CAD build for the part. Positions are in the model's coordinates, mm. Coordinates: 2 decimals unless noted, no trailing zeros. Write each loop counter-clockwise with the first axis right and the second up, starting at its lowest first coordinate (ties: lowest second). Pieces come first, ordered by that corner, then holes. Notation, with made-up numbers: (42.25, 50.25) - (89.25, 50.25) arc R18 cw to (89.25, 85.25) - close; hole circle Ø4 at (-29.5, -27.5). An arc over 180 degrees is marked (long way). One line per question, with ' | ' between items. Start each with the question number.
1. Band-saw the part on D-D, the plane z = -5.5. Write the cut outline in (x, y), then the cut area to 3 significant figures.
2. Flat gauge pins, fed straight in: P1, Ø5.5, axis at y = 97.47, z = 3.94, coming from the +X side; P2, Ø1.5, axis at x = 30.5, z = -56, coming from the +Y side; P3, Ø1.5, axis at x = 30.5, y = 98, coming from the +Z side; P4, Ø10, axis at y = 125.5, z = -1, coming from the +X side. Where does each tip first touch, or does it go through?
3. Band-saw the part on A-A, the plane y = 42. Write the cut outline in (x, z).
4. Band-saw the part on C-C, the plane z = -22.5. Write the cut outline in (x, y), then the cut area to 3 significant figures.
5. Two-plate mould, pull along Z, no slides. Class faces 1 (the cylindrical face through (29.786, 108.104, -65.421)), 2 (the cylindrical face through (30.48, 139.74, -30.23)), 3 (the flat face through (30.48, 131, -54.37)): +Z half, -Z half, draft (parallel to the pull), parting line (faces both ways), or undercut.
6. Probe line 1 (Z direction, x = 29.4, y = 42); line 2 (Z direction, x = 30.9, y = 85); line 3 (Y direction, x = 29.45, z = 22.5). List the from-to ranges inside material, lowest first.
7. Band-saw the part on B-B, the plane x = 29.6. Give the number of separate pieces and of enclosed holes in the cut face, then the cut area to 3 significant figures.
from build123d import *

# Parameters (mm, degrees)
BOSS_EXTRUDE1_DEPTH                            = 3
CSK_FOR_M3_FLAT_HEAD_MACHINE_SCREW1_AT_2_COUNT = 2
CSK_FOR_M3_FLAT_HEAD_MACHINE_SCREW1_AT_2_PITCH = 24.36335345
CSK_FOR_M3_FLAT_HEAD_MACHINE_SCREW1_AT_3_COUNT = 2
CSK_FOR_M3_FLAT_HEAD_MACHINE_SCREW1_AT_3_PITCH = 69.5
CSK_FOR_M3_FLAT_HEAD_MACHINE_SCREW1_AT_4_COUNT = 2
CSK_FOR_M3_FLAT_HEAD_MACHINE_SCREW1_AT_4_PITCH = 73.646608824
CSK_FOR_M3_FLAT_HEAD_MACHINE_SCREW1_AT_5_COUNT = 2
CSK_FOR_M3_FLAT_HEAD_MACHINE_SCREW1_AT_5_PITCH = 56.579922425
CSK_FOR_M3_FLAT_HEAD_MACHINE_SCREW1_AT_6_COUNT = 2
CSK_FOR_M3_FLAT_HEAD_MACHINE_SCREW1_AT_6_PITCH = 38.581652039
CSK_FOR_M3_FLAT_HEAD_MACHINE_SCREW1_AT_7_COUNT = 2
CSK_FOR_M3_FLAT_HEAD_MACHINE_SCREW1_AT_7_PITCH = 110.143173396
CSK_FOR_M3_FLAT_HEAD_MACHINE_SCREW1_AT_8_COUNT = 2
CSK_FOR_M3_FLAT_HEAD_MACHINE_SCREW1_AT_8_PITCH = 79.535664399


with BuildPart() as part:
    # Sketch2 → Boss-Extrude1 (new body)
    with BuildSketch(Plane(origin=(29, 0, 0), x_dir=(0, 0, -1), z_dir=(1, 0, 0))):
        with BuildLine():
            Line((-16.691511003, 108.816260881), (16.610141275, 134.506640075))
            ThreePointArc((16.610141275, 134.506640075), (30.439693581, 139.756494337), (44.856843921, 136.445412513))
            Line((44.856843921, 136.445412513), (64.147238229, 125.399811115))
            ThreePointArc((64.147238229, 125.399811115), (67.359474123, 122.47213667), (69.026291478, 118.458228724))
            Line((69.026291478, 118.458228724), (76.03531425, 78.708085309))
            ThreePointArc((76.03531425, 78.708085309), (75.841855651, 74.366160521), (73.824664919, 70.516397068))
            Line((73.824664919, 70.516397068), (59.475441909, 53.539223516))
            ThreePointArc((59.475441909, 53.539223516), (55.128189361, 49.472265428), (49.95644752, 46.524072909))
            Line((49.95644752, 46.524072909), (27.5, 37))
            Line((27.5, 37), (-27.5, 37))
            Line((-27.5, 37), (-42.183846688, 39.106824497))
            ThreePointArc((-42.183846688, 39.106824497), (-52.615538646, 44.799981854), (-56.769427994, 55.934497609))
            Line((-56.769427994, 55.934497609), (-56.769427994, 88.583208534))
            ThreePointArc((-56.769427994, 88.583208534), (-53.260094641, 98.225022679), (-44.374150659, 103.355324829))
            Line((-44.374150659, 103.355324829), (-18.877327121, 107.851102741))
            ThreePointArc((-18.877327121, 107.851102741), (-17.725917606, 108.201192201), (-16.691511003, 108.816260881))
        make_face()
    extrude(amount=BOSS_EXTRUDE1_DEPTH)

    # Sketch4 → CSK for M3 Flat Head Machine Screw1 (revolve, cut)
    with BuildSketch(Plane(origin=(32, 109.537877634, -64.506630382), x_dir=(0, 0, -1), z_dir=(0, 1, 0))):
        Polygon((0, 0), (0, 3), (1.7, 3), (1.7, 1.45), (3.15, 0), align=None)
    csk_for_m3_flat_head_machine_screw1 = revolve(axis=Axis((38.35, 109.537877634, -64.506630382), (-1, 0, 0)), mode=Mode.SUBTRACT)

    # CSK for M3 Flat Head Machine Screw1 at 2: CSK for M3 Flat Head Machine Screw1 ×2
    with Locations(*[Vector(0, -0.984807753, -0.173648178) * (i * CSK_FOR_M3_FLAT_HEAD_MACHINE_SCREW1_AT_2_PITCH) for i in range(1, CSK_FOR_M3_FLAT_HEAD_MACHINE_SCREW1_AT_2_COUNT)]):
        add(csk_for_m3_flat_head_machine_screw1, mode=Mode.SUBTRACT)

    # CSK for M3 Flat Head Machine Screw1 at 3: CSK for M3 Flat Head Machine Screw1 ×2
    with Locations(*[Vector(0, -0.173648178, 0.984807753) * (i * CSK_FOR_M3_FLAT_HEAD_MACHINE_SCREW1_AT_3_PITCH) for i in range(1, CSK_FOR_M3_FLAT_HEAD_MACHINE_SCREW1_AT_3_COUNT)]):
        add(csk_for_m3_flat_head_machine_screw1, mode=Mode.SUBTRACT)

    # CSK for M3 Flat Head Machine Screw1 at 4: CSK for M3 Flat Head Machine Screw1 ×2
    with Locations(*[Vector(0, -0.489659582, 0.871913696) * (i * CSK_FOR_M3_FLAT_HEAD_MACHINE_SCREW1_AT_4_PITCH) for i in range(1, CSK_FOR_M3_FLAT_HEAD_MACHINE_SCREW1_AT_4_COUNT)]):
        add(csk_for_m3_flat_head_machine_screw1, mode=Mode.SUBTRACT)

    # CSK for M3 Flat Head Machine Screw1 at 5: CSK for M3 Flat Head Machine Screw1 ×2
    with Locations(*[Vector(0, -0.918977854, 0.394309147) * (i * CSK_FOR_M3_FLAT_HEAD_MACHINE_SCREW1_AT_5_PITCH) for i in range(1, CSK_FOR_M3_FLAT_HEAD_MACHINE_SCREW1_AT_5_COUNT)]):
        add(csk_for_m3_flat_head_machine_screw1, mode=Mode.SUBTRACT)

    # CSK for M3 Flat Head Machine Screw1 at 6: CSK for M3 Flat Head Machine Screw1 ×2
    with Locations(*[Vector(0, 0.446748348, 0.894659663) * (i * CSK_FOR_M3_FLAT_HEAD_MACHINE_SCREW1_AT_6_PITCH) for i in range(1, CSK_FOR_M3_FLAT_HEAD_MACHINE_SCREW1_AT_6_COUNT)]):
        add(csk_for_m3_flat_head_machine_screw1, mode=Mode.SUBTRACT)

    # CSK for M3 Flat Head Machine Screw1 at 7: CSK for M3 Flat Head Machine Screw1 ×2
    with Locations(*[Vector(0, -0.613182602, 0.789941198) * (i * CSK_FOR_M3_FLAT_HEAD_MACHINE_SCREW1_AT_7_PITCH) for i in range(1, CSK_FOR_M3_FLAT_HEAD_MACHINE_SCREW1_AT_7_COUNT)]):
        add(csk_for_m3_flat_head_machine_screw1, mode=Mode.SUBTRACT)

    # CSK for M3 Flat Head Machine Screw1 at 8: CSK for M3 Flat Head Machine Screw1 ×2
    with Locations(*[Vector(0, -0.849152115, 0.528148356) * (i * CSK_FOR_M3_FLAT_HEAD_MACHINE_SCREW1_AT_8_PITCH) for i in range(1, CSK_FOR_M3_FLAT_HEAD_MACHINE_SCREW1_AT_8_COUNT)]):
        add(csk_for_m3_flat_head_machine_screw1, mode=Mode.SUBTRACT)


solid = part.part
Filled in:
1) outline: (29, 37) - (32, 37) - (32, 125.94) - (29, 125.94) - close | area: 267 mm²
2) P1: stops at x = 31.6 | P2: stops at y = 130.49 | P3: stops at z = 54.01 | P4: stops at x = 32
3) outline: (29, -39.29) - (32, -39.29) - (32, -25.65) - (30.55, -24.2) - (29, -24.2) - close; (29, -20.8) - (30.55, -20.8) - (32, -19.35) - (32, 19.35) - (30.55, 20.8) - (29, 20.8) - close; (29, 24.2) - (30.55, 24.2) - (32, 25.65) - (32, 49.51) - (29, 49.51) - close
4) outline: (29, 37) - (32, 37) - (32, 38.85) - (30.55, 40.3) - (29, 40.3) - close; (29, 43.7) - (30.55, 43.7) - (32, 45.15) - (32, 137.91) - (29, 137.91) - close | area: 290 mm²
5) face 1: undercut | face 2: parting line | face 3: -Z half
6) line 1: z = -39.29 to -24.2, -20.8 to 20.8, 24.2 to 49.51 | line 2: z = -74.93 to -70.71, -66.76 to 56.77 | line 3: y = 37 to 40.3, 43.7 to 107.21
7) separate pieces: 1 | enclosed holes: 8 | area: 10,200 mm²
